The figure shows three views and two pictorial views of one solid part (mm, origin at its lowest corner). Answer the questions. A direction names the side the tool comes from. Round coordinates to 2 decimals unless told otherwise and drop trailing zeros. Write each loop counter-clockwise with the first axis right and the second up, starting at its lowest first coordinate (ties: lowest second). Pieces come first, ordered by that corner, then holes. Notation, with made-up numbers: M 83.5,36.25 L 127.5,36.25 A9 ccw 127.5,53.25 Z; hole C -39,86 d2. An arc over 180 degrees is marked long. One line per item, written item: value. Start each with the question number.
Q1. The mould has two halves that part along Y. Classify the marked faces 1, 2, 3 and 4: released by +Y, released by -Y, zero draft, split by the parting line, or undercut.
Q2. Consider probe 1 along X at (y, z) = (11.75, 6); probe 2 along Y at (x, z) = (3.5, 1); probe 3 along Y at (x, z) = (28, 1). Determine where each line is inside the solid, lowest interval first.
Q3. Find section C-C (y = 4.75). Write down the section's boundary in (x, z), and give its area (3 significant figures).
Q4. A tool of negligible diameter and unlimited length cuts with its end or side. For the marked faces 5, 6, 7, 8 and 9, from which of +Z, -Z, +X, -X, +Y, -Y can it reach the whole face along a straight path? Write none if from no direction.
Q5. Find section B-B (x = 5). Write down the section's boundary in (y, z), and give its area (3 significant figures).
Q6. Given pin 1 Ø4 at (y, z) = (7, 2.5) entering from -X; pin 2 Ø2.5 at (y, z) = (5, 7) entering from -X, each flat-ended and moving along its own axis, determine where each tip first touches the part or whether it passes through.
Q7. Find section A-A (y = 10.5). Write down the section's boundary in (x, z).
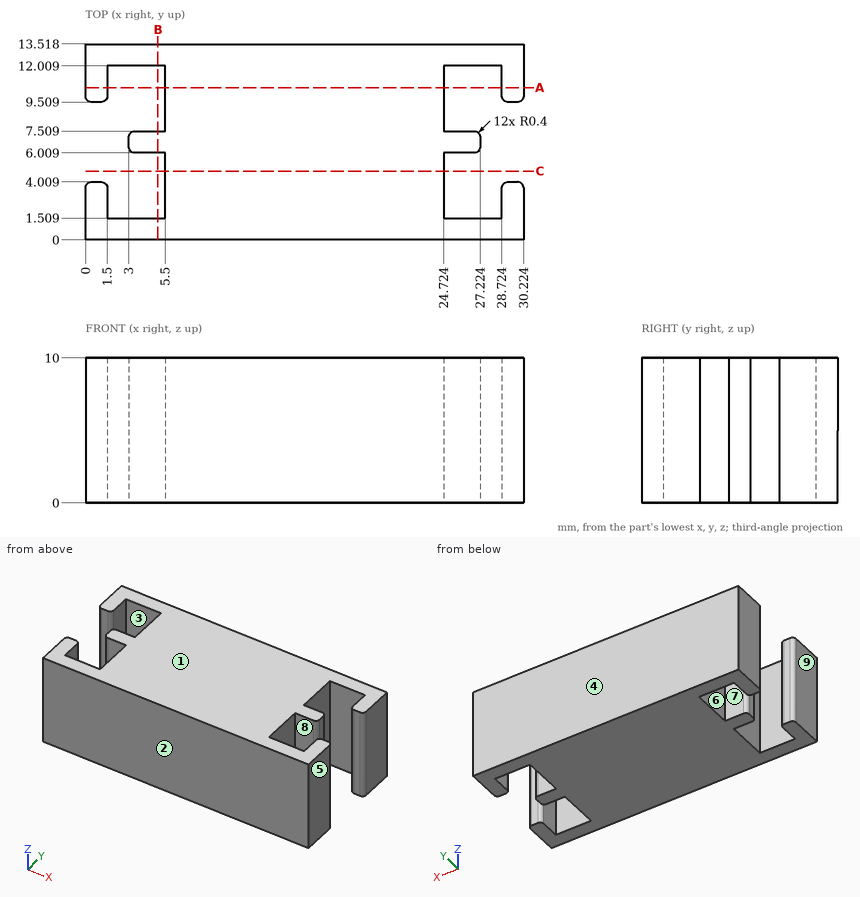
The answers:
1. face 1: zero draft
1. face 2: released by -Y
1. face 3: undercut
1. face 4: released by +Y
2. probe 1: 0 to 1.5, 5.5 to 24.72, 28.72 to 30.22
2. probe 2: 0 to 1.51, 6.01 to 7.51, 12.01 to 13.52
2. probe 3: 0 to 1.51, 12.01 to 13.52
3. outline: M 5.5,0 L 24.72,0 L 24.72,10 L 5.5,10 Z
3. area: 192 mm2
4. face 5: +Z, -Z, +X, +Y, -Y
4. face 6: +Z, -Z
4. face 7: +Z, -Z, -X
4. face 8: +Z, -Z, +X
4. face 9: +Z, -Z, -X, +Y, -Y
5. outline: M 0,0 L 1.51,0 L 1.51,10 L 0,10 Z; M 6.01,0 L 7.51,0 L 7.51,10 L 6.01,10 Z; M 12.01,0 L 13.52,0 L 13.52,10 L 12.01,10 Z
5. area: 45.2 mm2
6. pin 1: x = 3
6. pin 2: x = 0.03
7. outline: M 0,0 L 1.5,0 L 1.5,10 L 0,10 Z; M 5.5,0 L 24.72,0 L 24.72,10 L 5.5,10 Z; M 28.72,0 L 30.22,0 L 30.22,10 L 28.72,10 Z
